Here's how the part is built. I have some questions about the finished solid (model axes, mm). Face numbers are marked on the shaded views. A direction names the side the tool comes from. Give positions to 0.01 mm unless a question says otherwise; leave off trailing zeros. Loops run counter-clockwise (first coordinate to the right, second up) from the corner with the lowest first, then second, coordinate; pieces in that order, holes last.
Q1. I'm going to push flat-ended pins straight in: P1, Ø1, axis at x = 23.5, z = 6.5, coming from the +Y side; P2, Ø8, axis at x = 31, z = 13, coming from the +Y side; P3, Ø10, axis at y = 59, z = 11.5, coming from the +X side. Where does each tip first touch, or does it pass through?
Q2. For the marked faces 4 and 5, which set-ups out of +Z, -Z, +X, -X, +Y, -Y let a thin tool reach every point of the face, with its end or its side?
Q3. I need wall thicknesses on probe 1 along Y at (x, z) = (35, 8.5); probe 2 along X at (y, z) = (54.5, 1.5); probe 3 along Y at (x, z) = (32, 3.25). Which ranges of each line are inside material? Lowest first, please.
Q4. Thinking about a two-plate mould opening in Y: for the marked faces 1, 2 and 3, which applies, pulls with the +Y half, pulls with the -Y half, needs draft (parallel to the pull), parting line crosses it, or undercut?
Q5. Suppose I cut it at B-B (y = 20). List the corners of the cut face in (x, z) for me, and give its area (3 significant figures).
Q6. Suppose I cut it at A-A (z = 10). List the corners of the cut face in (x, y) for me, and give its area (3 significant figures).
Q7. Suppose I cut it at D-D (z = 2). List the corners of the cut face in (x, y) for me, and give its area (3 significant figures).
Q8. Suppose I cut it at C-C (x = 32.5). List the corners of the cut face in (y, z) for me, and give its area (3 significant figures).
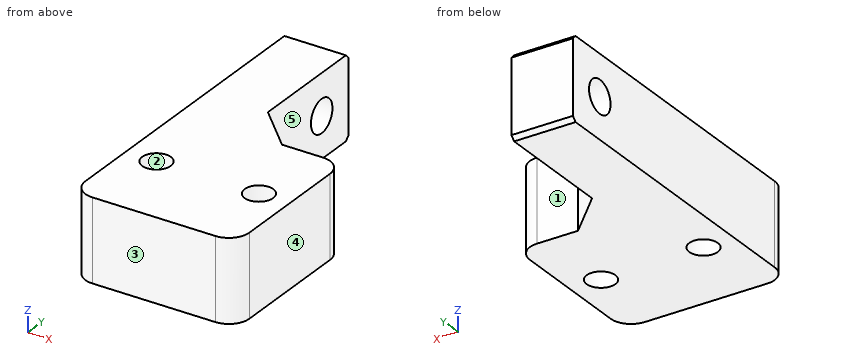
```python
from build123d import *

# Parameters (mm, degrees)
ESQUISSE1_W                  = 40
ESQUISSE1_H                  = 40
BOSS_EXTRU_1_DEPTH           = 20
ESQUISSE2_W                  = 15
ESQUISSE2_H                  = 40
BOSS_EXTRU_2_DEPTH           = 20
ENL_V_MAT_EXTRU_1_DEPTH      = 92.651513899
ENL_V_MAT_EXTRU_1_DEPTH_BACK = 92.651513899
ESQUISSE3_R                  = 3.5
ENL_V_MAT_EXTRU_2_DEPTH      = 92.651513899
ENL_V_MAT_EXTRU_2_DEPTH_BACK = 92.651513899
ESQUISSE4_R                  = 4
CONG_1_R                     = 5
CHANFREIN1_SIZE              = 10
CHANFREIN2_SIZE              = 1


with BuildPart() as part:
    # Esquisse1 → Boss.-Extru.1 (new body)
    with BuildSketch(Plane.XY):
        with Locations((20, 20)):
            Rectangle(ESQUISSE1_W, ESQUISSE1_H)
    extrude(amount=BOSS_EXTRU_1_DEPTH)

    # Esquisse2 → Boss.-Extru.2 (add)
    with BuildSketch(Plane.XY.offset(20)):
        with Locations((7.5, 60)):
            Rectangle(ESQUISSE2_W, ESQUISSE2_H)
    extrude(amount=-BOSS_EXTRU_2_DEPTH)

    # Esquisse3 → Enlèv. mat.-Extru.1 (cut, two sides: drawn at the far end of the back side and taken through both)
    with BuildSketch(Plane.XY.offset(20).offset(-ENL_V_MAT_EXTRU_1_DEPTH_BACK)):
        with Locations((7.5, 20)):
            Circle(ESQUISSE3_R)
        with Locations(Location((32.5, 20, 0), (0, 0, 180))):
            Circle(ESQUISSE3_R)
    extrude(amount=ENL_V_MAT_EXTRU_1_DEPTH + ENL_V_MAT_EXTRU_1_DEPTH_BACK, mode=Mode.SUBTRACT)

    # Esquisse4 → Enlèv. mat.-Extru.2 (cut, two sides: drawn at the far end of the back side and taken through both)
    with BuildSketch(Plane.ZY.offset(-ENL_V_MAT_EXTRU_2_DEPTH_BACK)):
        with Locations(Location((10, 70, 0), (0, 0, 180))):
            Circle(ESQUISSE4_R)
    extrude(amount=ENL_V_MAT_EXTRU_2_DEPTH + ENL_V_MAT_EXTRU_2_DEPTH_BACK, mode=Mode.SUBTRACT)

    # Congé1
    cong_1_edges = [part.edges().sort_by_distance(p)[0] for p in [
        (40, 40, 10),
        (40, 0, 10),
        (0, 0, 10),
    ]]
    fillet(cong_1_edges, radius=CONG_1_R)

    # Chanfrein1
    chanfrein1_edges = [part.edges().sort_by_distance(p)[0] for p in [
        (15, 40, 10),
    ]]
    chamfer(chanfrein1_edges, length=CHANFREIN1_SIZE)

    # Chanfrein2
    chanfrein2_edges = [part.edges().sort_by_distance(p)[0] for p in [
        (7.5, 80, 0),
        (7.5, 80, 20),
    ]]
    chamfer(chanfrein2_edges, length=CHANFREIN2_SIZE)


solid = part.part
```
Solutions:
1. P1: stops at y = 42
1. P2: stops at y = 40
1. P3: stops at x = 15
2. face 4: +Z, -Z, +X, +Y, -Y
2. face 5: +Z, -Z, +X, +Y
3. probe 1: y = 0 to 17.55, 22.45 to 40
3. probe 2: x = 0 to 15
3. probe 3: y = 0 to 16.54, 23.46 to 40
4. face 1: pulls with the +Y half
4. face 2: undercut
4. face 3: pulls with the -Y half
5. outline: (0, 0) - (4, 0) - (4, 20) - (0, 20) - close; (11, 0) - (29, 0) - (29, 20) - (11, 20) - close; (36, 0) - (40, 0) - (40, 20) - (36, 20) - close
5. area: 520 mm2
6. outline: (0, 5) arc R5 ccw to (5, 0) - (35, 0) arc R5 ccw to (40, 5) - (40, 35) arc R5 ccw to (35, 40) - (25, 40) - (15, 50) - (15, 66) - (0, 66) - close; (0, 74) - (15, 74) - (15, 80) - (0, 80) - close; hole circle Ø7 at (7.5, 20); hole circle Ø7 at (32.5, 20)
6. area: 2,040 mm2
7. outline: (0, 5) arc R5 ccw to (5, 0) - (35, 0) arc R5 ccw to (40, 5) - (40, 35) arc R5 ccw to (35, 40) - (25, 40) - (15, 50) - (15, 80) - (0, 80) - close; hole circle Ø7 at (7.5, 20); hole circle Ø7 at (32.5, 20)
7. area: 2,160 mm2
8. outline: (0, 0) - (16.5, 0) - (16.5, 20) - (0, 20) - close; (23.5, 0) - (40, 0) - (40, 20) - (23.5, 20) - close
8. area: 660 mm2
